Autodesk Inventor part; units mm, degrees
ref_plane "YZ Plane" through (0, 0, 0) normal (1, 0, 0) x (0, 1, 0)
ref_plane "XZ Plane" through (0, 0, 0) normal (0, 1, 0) x (-1, 0, 0)
ref_plane "XY Plane" through (0, 0, 0) normal (0, 0, 1) x (1, 0, 0)
sketch "Sketch2" plane through (0, 0, 0) normal (0, 0, 1) x (1, 0, 0)
  line L0 (0, 0) -> (42, 0)
  line L1 (42, 0) -> (42, 32)
  line L2 (42, 32) -> (0, 32)
  line L3 (0, 32) -> (0, 0)
  dimension "d0" = 42
  dimension "d1" = 32
extrude "Cover_Body" add sketch "Sketch2" along normal blind 15.8
sketch "Sketch4" plane through (0, 0, 15.8) normal (0, 0, 1) x (1, 0, 0)
  line L0 (42, 32) -> (0, 32)
  line L1 (0, 32) -> (0, 0)
  line L2 (4.5, 24.6) -> (9.5, 24.6)
  line L3 (32.5, 24.6) -> (37.5, 24.6)
  line L4 (42, 0) -> (42, 32)
  line L5 (0, 0) -> (42, 0)
  line L6 (4.5, 24.6) -> (4.5, 27.1)
  line L7 (4.5, 27.1) -> (9.5, 27.1)
  line L8 (9.5, 27.1) -> (9.5, 32)
  line L9 (37.5, 27.1) -> (37.5, 24.6)
  line L10 (37.5, 27.1) -> (32.5, 27.1)
  line L11 (32.5, 27.1) -> (32.5, 32)
  line L12 (9.5, 32) -> (32.5, 32)
  line L13 (21, 36.5125) -> (21, -47.625) construction
  line L14 (32.5, 24.6) -> (32.5, 0)
  line L15 (9.5, 24.6) -> (9.5, 0)
  line L16 (9.5, 0) -> (32.5, 0)
  point P0 (4.9935, 32)
  point P1 (37, 32)
  dimension "d6" = 5
  dimension "d14" = 2.5
  dimension "d15" = 2.5
  dimension "d22" = 42
  dimension "d23" = 21
  dimension "d24" = 23
  dimension "d28" = 5
  dimension "d118" = 23
  dimension "d119" = 11.5
  dimension "d120" = 11.5
  dimension "d121" = 24.6
extrude "Servo_Opening" cut sketch "Sketch4" against normal blind 6.3 contours L11 L10 L9 L3 L14 L5 L15 L2 L6 L7 L8 L0
sketch "Sketch5" plane through (0, 0, 15.8) normal (0, 0, 1) x (1, 0, 0)
  line L0 (0, 32) -> (0, 0)
  line L1 (0, 13.2) -> (0, 14.7)
  line L2 (-29.647, 13.95) -> (54.8226, 13.95) construction
  line L3 (0, 0) -> (42, 0)
  line L4 (0, 14.7) -> (9.5, 14.7)
  line L5 (9.5, 14.7) -> (9.5, 13.2)
  line L6 (9.5, 13.2) -> (0, 13.2)
  line L7 (9.5, 0) -> (9.5, 24.6)
  line L8 (9.5, 32) -> (0, 32)
  dimension "d97" = 1.5
  dimension "d131" = 13.2
extrude "Cable_Opening" cut sketch "Sketch5" against normal blind 2.5 contours L4 L5 L6 L0
sketch "Sketch6" plane through (0, 0, 15.8) normal (0, 0, 1) x (1, 0, 0)
  circle A0 centre (3.5, 28) radius 1.25
  circle A1 centre (38.5, 28) radius 1.25 construction
  circle A2 centre (38.5, 4) radius 1.25
  circle A3 centre (3.5, 4) radius 1.25 construction
  line L0 (21, 34.35) -> (21, -13.275) construction
  line L1 (-20.6375, 16) -> (66.675, 16) construction
  line L2 (42, 0) -> (42, 32)
  line L3 (0, 32) -> (0, 0)
  line L4 (9.5, 32) -> (0, 32)
  line L5 (0, 0) -> (42, 0)
  point P0 (42, 12.35)
  point P1 (0, 12.35)
  dimension "d29" = 2.5
  dimension "d30" = 2.5
  dimension "d31" = 2.5
  dimension "d32" = 2.5
  dimension "d33" = 42
  dimension "d34" = 21
  dimension "d35" = 32
  dimension "d36" = 16
  dimension "d37" = 35
  dimension "d38" = 17.5
  dimension "d39" = 24
  dimension "d40" = 12
extrude "Holes_Mounting_Screws" cut sketch "Sketch6" against normal up to surface (15.8 mm away)
sketch "Sketch16" plane through (0, 0, 0) normal (0, 0, -1) x (-1, 0, 0)
  circle A0 centre (-38.5, 4) radius 2.25
  circle A1 centre (-3.5, 28) radius 2.25
  circle A2 centre (-38.5, 4) radius 1.25
  circle A3 centre (-3.5, 28) radius 1.25
  dimension "d99" = 4.5
  dimension "d100" = 4.5
extrude "Pocket_Mounting_Screws" cut sketch "Sketch16" against normal blind 9
sketch "Sketch17" plane through (0, 0, 9.5) normal (0, 0, 1) x (1, 0, 0)
  circle A0 centre (14.75, 26.6) radius 1.75
  line L0 (9.5, 32) -> (32.5, 32)
  line L1 (9.5, 27.1) -> (9.5, 32)
  point P0 (0, 0)
  dimension "d105" = 3.5
  dimension "d106" = 5.4
  dimension "d107" = 5.25
extrude "Heat_Dissipation_Hole" cut sketch "Sketch17" against normal up to surface (9.5 mm away)
pattern_linear "Pattern_Heat_Dissipation_Hole" count 3 spacing 6.25 along (1, 0, 0) count 3 spacing 6.25 along (0, -1, 0) of "Heat_Dissipation_Hole"
sketch "Sketch25" plane through (0, 0, 0) normal (0, 0, -1) x (-1, 0, 0)
  line L0 (0, 32) -> (0, 0)
  line L1 (-42, 32) -> (-32.5, 32)
  line L2 (0, 0) -> (-42, 0)
  line L3 (-42, 0) -> (-42, 32)
  line L4 (-42, 32) -> (0, 32)
  line L5 (0, 32) -> (0, 0)
extrude "Material_Reduction_Optional" cut sketch "Sketch25" against normal blind 1.5
equation "\"d15\" = d14"
equation "\"d23\" = 0.5 * d22"
equation "\"d28\" = d6"
equation "\"d120\" = 0.5 * d118"
equation "\"d34\" = 0.5 * d33"
equation "\"d36\" = 0.5 * d35"
equation "\"d38\" = 0.5 * d37"
equation "\"d40\" = 0.5 * d39"
equation "\"d99\" = d101"
equation "\"d100\" = d101"
properties part number "EDMO1-0_Cover" material "PLA"
Can you work these out from the model? Positions are in its coordinate system, mm. A direction names the side the tool comes from. Give positions to 0.01 mm unless a question says otherwise; leave off trailing zeros. Write each loop counter-clockwise with the first axis right and the second up, starting at its lowest first coordinate (ties: lowest second). Pieces come first, ordered by that corner, then holes. Notation, with made-up numbers: (79, -24.75) -> (104, -24.75) arc R13 ccw to (104, 0.25) -> close; hole circle Ø4 at (38, 82). An arc over 180 degrees is marked (long way). Answer as a JSON object with one key per item and string values. Group by question number.
Item 1: Suppose I cut it at A-A (x = 3.5). Please give me the cut outline in (y, z), plus the area to 3 significant figures.
Item 2: Please list where these lines run through material, in increasing order: line 1 (Y direction, x = 14.75, z = 4.5); line 2 (Y direction, x = 38.5, z = 12.5); line 3 (X direction, y = 12.5, z = 13.75). Write a range as [from, to].
Item 3: I'm going to push flat-ended pins straight in: P1, Ø7, axis at x = 3.5, y = 28, coming from the +Z side; P2, Ø6, axis at x = 17, y = 15, coming from the +Z side; P3, Ø1.3, axis at x = 3.5, y = 29, coming from the -Z side. Where does each tip first touch, or does it pass through?
Item 4: Suppose I cut it at C-C (z = 11.75). Please give me the cut outline in (x, y).
Item 5: Suppose I cut it at D-D (x = 14.75). Please give me the cut outline in (y, z).
Item 6: For faces 4 (the face through (37.5, 26, 13)), 5 (the face through (2.5, 27, 9)), 6 (the face through (5, 13.2, 15)), 7 (the face through (32.5, 30, 13)), 8 (the face through (19.6, 19.3, 5.6)), which set-ups out of +Z, -Z, +X, -X, +Y, -Y let a thin tool reach every point of the face, with its end or its side?
Item 7: Suppose I cut it at B-B (y = 4). Please give me the cut outline in (x, z).
Item 8: We'd pull the mould along X, two halves only. Please class faces 1 (the face through (21, 0, 7)), 2 (the face through (2.462, 26.004, 5.198)), 3 (the face through (42, 16, 9)): +X half, -X half, draft (parallel to the pull), parting line (faces both ways), or undercut.
Findings:
{
 "1": {"outline": "(0, 1.5) -> (25.75, 1.5) -> (25.75, 9) -> (26.75, 9) -> (26.75, 15.8) -> (14.7, 15.8) -> (14.7, 13.3) -> (13.2, 13.3) -> (13.2, 15.8) -> (0, 15.8) -> close; (29.25, 9) -> (30.25, 9) -> (30.25, 1.5) -> (32, 1.5) -> (32, 15.8) -> (29.25, 15.8) -> close", "area": "403 mm²"},
 "2": {"line 1": "y = [0, 12.35], [15.85, 18.6], [22.1, 24.85], [28.35, 32]", "line 2": "y = [0, 2.75], [5.25, 32]", "line 3": "x = [0, 9.5], [32.5, 42]"},
 "3": {"P1": "stops at z = 15.8", "P2": "stops at z = 9.5", "P3": "stops at z = 9"},
 "4": {"outline": "(0, 0) -> (9.5, 0) -> (9.5, 24.6) -> (4.5, 24.6) -> (4.5, 27.1) -> (9.5, 27.1) -> (9.5, 32) -> (0, 32) -> close; (32.5, 0) -> (42, 0) -> (42, 32) -> (32.5, 32) -> (32.5, 27.1) -> (37.5, 27.1) -> (37.5, 24.6) -> (32.5, 24.6) -> close; hole circle Ø2.5 at (3.5, 28); hole circle Ø2.5 at (38.5, 4)"},
 "5": {"outline": "(0, 1.5) -> (12.35, 1.5) -> (12.35, 9.5) -> (0, 9.5) -> close; (15.85, 1.5) -> (18.6, 1.5) -> (18.6, 9.5) -> (15.85, 9.5) -> close; (22.1, 1.5) -> (24.85, 1.5) -> (24.85, 9.5) -> (22.1, 9.5) -> close; (28.35, 1.5) -> (32, 1.5) -> (32, 9.5) -> (28.35, 9.5) -> close"},
 "6": {"face 4": "+Z", "face 5": "-Z", "face 6": "+Z, -X", "face 7": "+Z, +Y, -Y", "face 8": "+Z, -Z"},
 "7": {"outline": "(0, 1.5) -> (36.25, 1.5) -> (36.25, 9) -> (37.25, 9) -> (37.25, 15.8) -> (32.5, 15.8) -> (32.5, 9.5) -> (9.5, 9.5) -> (9.5, 15.8) -> (0, 15.8) -> close; (39.75, 9) -> (40.75, 9) -> (40.75, 1.5) -> (42, 1.5) -> (42, 15.8) -> (39.75, 15.8) -> close"},
 "8": {"face 1": "draft", "face 2": "undercut", "face 3": "+X half"}
}
